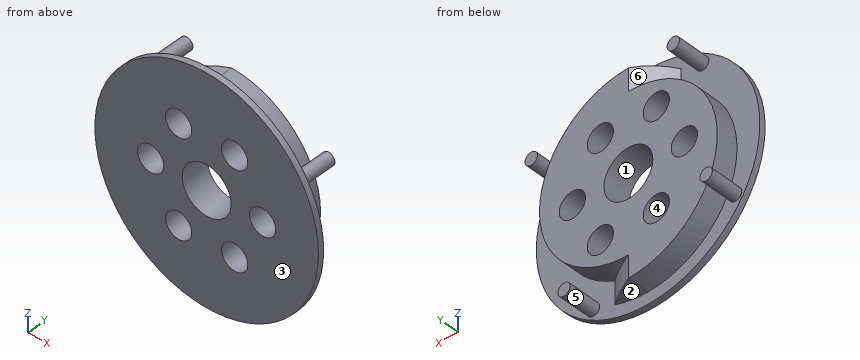
from build123d import *

# Parameters (mm, degrees)
SKETCH1_R          = 63.881
EXTRUDE1_DEPTH     = 3.302
EXTRUDE2_DEPTH     = 12.446
SKETCH5_R          = 13.97
CUT_EXTRUDE3_DEPTH = 16.748
SKETCH7_R          = 7.493
CUT_EXTRUDE4_DEPTH = 16.748
CIRPATTERN1_COUNT  = 6
EXTRUDE3_START     = 40.844813
EXTRUDE3_DEPTH     = 16.305187
CUT_EXTRUDE5_DEPTH = 12.446
EXTRUDE4_START     = -57.15
EXTRUDE4_DEPTH     = 16.305187
CUT_EXTRUDE6_DEPTH = 12.446
SKETCH22_R         = 3.556
EXTRUDE5_DEPTH     = 18.542
CIRPATTERN2_COUNT  = 4


with BuildPart() as part:
    # Sketch1 → Extrude1 (new body)
    with BuildSketch(Plane(origin=(0, 0, 0), x_dir=(1, 0, 0), z_dir=(0, 1, 0))):
        Circle(SKETCH1_R)
    extrude(amount=EXTRUDE1_DEPTH)

    # Sketch4 → Extrude2 (add)
    with BuildSketch(Plane(origin=(0, 3.302, 0), x_dir=(-1, 0, 0), z_dir=(0, 1, 0))):
        with BuildLine():
            Line((0, -57.15), (0, -44.45))
            ThreePointArc((0, -44.45), (-50.8, 6.35), (0, 57.15))
            Line((0, 57.15), (0, 44.45))
            ThreePointArc((0, 44.45), (50.8, -6.35), (0, -57.15))
        make_face()
    extrude(amount=EXTRUDE2_DEPTH)

    # Sketch5 → Cut-Extrude3 (cut, through all)
    with BuildSketch(Plane(origin=(0, 15.748, 0), x_dir=(-1, 0, 0), z_dir=(0, 1, 0))):
        Circle(SKETCH5_R)
    extrude(amount=-CUT_EXTRUDE3_DEPTH, mode=Mode.SUBTRACT)

    # Sketch7 → Cut-Extrude4 (cut, through all)
    with BuildSketch(Plane(origin=(0, 15.748, 0), x_dir=(-1, 0, 0), z_dir=(0, 1, 0))):
        with Locations((-32.004, 0)):
            Circle(SKETCH7_R)
    cut_extrude4 = extrude(amount=-CUT_EXTRUDE4_DEPTH, mode=Mode.SUBTRACT)

    # CirPattern1: Cut-Extrude4 ×6 about axis
    cirpattern1_axis = Axis((0, 0, 0), (0, 1, 0))
    for i in range(1, CIRPATTERN1_COUNT):
        add(cut_extrude4.rotate(cirpattern1_axis, i * 360 / CIRPATTERN1_COUNT), mode=Mode.SUBTRACT)

    # Sketch18 → Extrude3 (add)
    with BuildSketch(Plane.XY.offset(EXTRUDE3_START)):
        with BuildLine():
            Line((0, 3.302), (-18.796, 3.302))
            ThreePointArc((-18.796, 3.302), (-9.88893997, 10.266419547), (0, 15.748))
            Line((0, 15.748), (0, 3.302))
        make_face()
    extrude(amount=EXTRUDE3_DEPTH)

    # Sketch19 → Cut-Extrude5 (cut)
    with BuildSketch(Plane(origin=(0, 15.748, 0), x_dir=(-1, 0, 0), z_dir=(0, 1, 0))):
        with BuildLine():
            Line((18.796, 53.970666885), (18.796, 57.15))
            Line((18.796, 57.15), (0, 57.15))
            ThreePointArc((0, 57.15), (9.531497457, 56.349561278), (18.796, 53.970666885))
        make_face()
    extrude(amount=-CUT_EXTRUDE5_DEPTH, mode=Mode.SUBTRACT)

    # Sketch20 → Extrude4 (add)
    with BuildSketch(Plane.XY.offset(EXTRUDE4_START)):
        with BuildLine():
            Line((0, 3.302), (18.796, 3.302))
            ThreePointArc((18.796, 3.302), (9.88893997, 10.266419547), (0, 15.748))
            Line((0, 15.748), (0, 3.302))
        make_face()
    extrude(amount=EXTRUDE4_DEPTH)

    # Sketch21 → Cut-Extrude6 (cut)
    with BuildSketch(Plane(origin=(0, 15.748, 0), x_dir=(-1, 0, 0), z_dir=(0, 1, 0))):
        with BuildLine():
            Line((0, -57.15), (-18.796, -57.15))
            Line((-18.796, -57.15), (-18.796, -53.970666885))
            ThreePointArc((-18.796, -53.970666885), (-9.531497457, -56.349561278), (0, -57.15))
        make_face()
    extrude(amount=-CUT_EXTRUDE6_DEPTH, mode=Mode.SUBTRACT)

    # Sketch22 → Extrude5 (add)
    with BuildSketch(Plane(origin=(0, 3.302, 57.15), x_dir=(1, 0, 0), z_dir=(0, -1, 0))):
        with Locations((49.97377821, -25.922917597)):
            Circle(SKETCH22_R)
    extrude5 = extrude(amount=-EXTRUDE5_DEPTH)

    # CirPattern2: Extrude5 ×4 about axis
    cirpattern2_axis = Axis((0, 0, 0), (0, 1, 0))
    for i in range(1, CIRPATTERN2_COUNT):
        add(extrude5.rotate(cirpattern2_axis, i * 360 / CIRPATTERN2_COUNT))


solid = part.part
CAD build for the part. Positions are in the model's coordinates, mm. Face numbers are marked on the shaded views. A direction names the side the tool comes from. Give positions to 0.01 mm unless a question says otherwise; leave off trailing zeros. Write each loop counter-clockwise with the first axis right and the second up, starting at its lowest first coordinate (ties: lowest second). Pieces come first, ordered by that corner, then holes. Notation, with made-up numbers: (67, -2.75) -> (110, -2.75) arc R17 ccw to (110, 13.25) -> close; hole circle Ø4 at (-12.5, 31.25). An arc over 180 degrees is marked (long way). Return JSON: item names as keys, results as strings.
Item 1: Band-saw the part on C-C (x = -1.5). List the corners of the cut face in (y, z).
Answer below:
{"outline": "(0, -63.86) -> (3.3, -63.86) -> (3.3, -57.13) -> (15.75, -57.13) -> (15.75, -13.89) -> (0, -13.89) -> close; (0, 13.89) -> (15.75, 13.89) -> (15.75, 44.43) -> (15.04, 44.43) -> (15.04, 57.13) -> (3.3, 57.13) -> (3.3, 63.86) -> (0, 63.86) -> close"}
Item 2: Drop flat-ended pins along their axis: pin 1 (17 mm diameter, centred on x = 16, z = -27.72, fed in from +Y); pin 2 (4 mm diameter, centred on x = -32.5, z = -48, fed in from -Y); pin 3 (8 mm diameter, centred on x = 9, y = 2.5, fed in from +Z) (3 decimals); pin 4 (1.5 mm diameter, centred on y = 18.5, z = -48.5, fed in from -X). Give the stop position or say it passes through.
Answer below:
{"pin 1": "stops at y = 15.75", "pin 2": "stops at y = 0", "pin 3": "stops at z = 63.685", "pin 4": "stops at x = 27.75"}
Item 3: Two-plate mould, pull along X, no slides. Class the marked faces 1, 2 and 3: +X half, -X half, draft (parallel to the pull), parting line (faces both ways), or undercut.
Answer below:
{"face 1": "undercut", "face 2": "+X half", "face 3": "draft"}
Item 4: Band-saw the part on B-B (z = 23). List the corners of the cut face in (x, y).
Answer below:
{"outline": "(-59.6, 0) -> (-21.82, 0) -> (-21.82, 15.75) -> (-41.46, 15.75) -> (-41.46, 3.3) -> (-59.6, 3.3) -> close; (-10.18, 0) -> (10.18, 0) -> (10.18, 15.75) -> (-10.18, 15.75) -> close; (21.82, 0) -> (59.6, 0) -> (59.6, 3.3) -> (47.99, 3.3) -> (47.99, 15.75) -> (21.82, 15.75) -> close"}
Item 5: Band-saw the part on D-D (z = 0). List the corners of the cut face in (x, y).
Answer below:
{"outline": "(-63.88, 0) -> (-39.5, 0) -> (-39.5, 15.75) -> (-50.4, 15.75) -> (-50.4, 3.3) -> (-63.88, 3.3) -> close; (-24.51, 0) -> (-13.97, 0) -> (-13.97, 15.75) -> (-24.51, 15.75) -> close; (13.97, 0) -> (24.51, 0) -> (24.51, 15.75) -> (13.97, 15.75) -> close; (39.5, 0) -> (63.88, 0) -> (63.88, 3.3) -> (50.4, 3.3) -> (50.4, 15.75) -> (39.5, 15.75) -> close"}
Item 6: Drill centre lines: probe 1 along X at (y, z) = (7, 0.5); probe 2 along Z at (x, y) = (15, 12.25); probe 3 along Z at (x, y) = (18.5, 1). Where is each one in solid material? Low to high.
Answer below:
{"probe 1": "x = -50.34 to -39.48, -24.53 to -13.96, 13.96 to 24.53, 39.48 to 50.46", "probe 2": "z = -42.18 to -35.14, -20.29 to 20.29, 35.14 to 54.88", "probe 3": "z = -61.14 to -34.78, -20.65 to 20.65, 34.78 to 61.14"}
Item 7: Tool access for the marked faces 4, 5 and 6: list every direction of +Z, -Z, +X, -X, +Y, -Y with a clear straight run to the whole face (end or side of a thin tool).
Answer below:
{"face 4": "+Y, -Y", "face 5": "+Y", "face 6": "+Z, +Y"}
Item 8: Band-saw the part on A-A (y = 9.25). Give the number of separate pieces and of enclosed holes in the cut face, then the cut area to 4 significant figures.
Answer below:
{"separate pieces": "5", "enclosed holes": "7", "area": "6,885 mm2"}
